from build123d import *

# Parameters (mm, degrees)
F0_R     = 27.5
F1_DEPTH = 10
F2_R     = 39.5
F3_DEPTH = 10
F4_R     = 27.5
F5_DEPTH = 30
F6_R     = 15
F7_DEPTH = 50.001
F9_D     = 6.6


with BuildPart() as f1:
    # F0 (on Top) → F1 (new body)
    with BuildSketch(Plane.XY):
        Circle(F0_R)
    extrude(amount=-F1_DEPTH)

    # F2 (on Top) → F3 (join)
    with BuildSketch(Plane.XY):
        Circle(F2_R)
    extrude(amount=F3_DEPTH)

    # F4 (on face) → F5 (join)
    with BuildSketch(Plane.XY.offset(10)):
        Circle(F4_R)
    extrude(amount=F5_DEPTH)

    # F6 (on face) → F7 (cut, through all)
    with BuildSketch(Plane.XY.offset(40)):
        Circle(F6_R)
    extrude(amount=-F7_DEPTH, mode=Mode.SUBTRACT)

    # F9 (through all)
    with Locations(Plane.XY.offset(10)):
        with Locations((0, 33.5), (33.5, 0), (0, -33.5), (-33.5, 0)):
            Hole(F9_D / 2)


solid = f1.part
Work out the finished part from the listing and answer in its coordinate system (mm). A direction names the side the tool comes from. Give positions to 0.01 mm unless a question says otherwise; leave off trailing zeros. Order: outer loops, then holes, each group sorted by start corner. A loop starts at its lowest first (then second) coordinate and runs counter-clockwise, first axis right, second up. Notation, with made-up numbers: (51, 64.5) - (71, 64.5) arc R29 cw to (71, 86.5) - close; hole circle Ø9 at (-34.75, 81). An arc over 180 degrees is marked (long way). Answer as CSV lines item,"result". Start each with the question number.
Q1. The part is cut by section C-C (z = 2.5). Write down the section's boundary in (x, y).
Q2. The part is cut by section D-D (x = -33.5). Write down the section's boundary in (y, z).
Q3. Given pin 1 Ø7.5 at (x, y) = (0, -33.5) entering from -Z; pin 2 Ø4 at (y, z) = (11, -1) entering from -X; pin 3 Ø4 at (x, z) = (9, 15) entering from -Y, each flat-ended and moving along its own axis, determine where each tip first touches the part or whether it passes through.
Q4. For faces 4 (the face through (-5.961, -26.846, 24.79)), 5 (the face through (12, -12, -10)), determine the directions among +Z, -Z, +X, -X, +Y, -Y from which every point of the face is accessible in a straight line to the end or side of a thin tool.
Q5. The part is cut by section A-A (x = 0). Write down the section's boundary in (y, z), then the cut area to 3 significant figures.
Q6. Find the intervals of material crossed by L1, parallel to Y at x = 0, z = 5; L2, parallel to Y at x = 0, z = 23; L3, parallel to Z at x = 31, y = 6.5, in increasing order. Write a range as [from, to].
Q7. The mould has two halves that part along Y. Classify faces 1 (the face through (-1.774, 36.283, 4.93)), 2 (the face through (-5.961, -26.846, -4.93)), 3 (the face through (-15, 24, 0)): +Y half, -Y half, draft (parallel to the pull), parting line (faces both ways), or undercut.
Check result:
1,outline,"circle Ø79 at (0, 0); hole circle Ø6.6 at (-33.5, 0); hole circle Ø30 at (0, 0); hole circle Ø6.6 at (0, -33.5); hole circle Ø6.6 at (0, 33.5); hole circle Ø6.6 at (33.5, 0)"
2,outline,"(-20.93, 0) - (-3.3, 0) - (-3.3, 10) - (-20.93, 10) - close; (3.3, 0) - (20.93, 0) - (20.93, 10) - (3.3, 10) - close"
3,pin 1,"stops at z = 0"
3,pin 2,"stops at x = -38.4"
3,pin 3,"stops at y = -26.59"
4,face 4,"+Z"
4,face 5,"-Z, +X, -X, +Y, -Y"
5,outline,"(-39.5, 0) - (-36.8, 0) - (-36.8, 10) - (-39.5, 10) - close; (-30.2, 0) - (-27.5, 0) - (-27.5, -10) - (-15, -10) - (-15, 40) - (-27.5, 40) - (-27.5, 10) - (-30.2, 10) - close; (15, -10) - (27.5, -10) - (27.5, 0) - (30.2, 0) - (30.2, 10) - (27.5, 10) - (27.5, 40) - (15, 40) - close; (36.8, 0) - (39.5, 0) - (39.5, 10) - (36.8, 10) - close"
5,area,"1,360 mm²"
6,L1,"y = [-39.5, -36.8], [-30.2, -15], [15, 30.2], [36.8, 39.5]"
6,L2,"y = [-27.5, -15], [15, 27.5]"
6,L3,"z = [0, 10]"
7,face 1,"undercut"
7,face 2,"parting line"
7,face 3,"draft"
